Here's how the part is built. I have some questions about the finished solid (model axes, mm). Face numbers are marked on the shaded views. A direction names the side the tool comes from. Give positions to 0.01 mm unless a question says otherwise; leave off trailing zeros. Write each loop counter-clockwise with the first axis right and the second up, starting at its lowest first coordinate (ties: lowest second). Pieces come first, ordered by that corner, then holes. Notation, with made-up numbers: (46, -11) - (69, -11) arc R22 cw to (69, 24) - close; hole circle Ø1 at (57.25, -18.5). An arc over 180 degrees is marked (long way). Write each question's results on one line, items separated by ' | '. Start each with the question number.
Item 1: Suppose I cut it at A-A on z = 0. List the corners of the cut face in (x, y) for me.
Item 2: Will these pins go through, and if not, where does the flat tip stop? P1, Ø2.5, axis at x = -38.89, z = -38.89, coming from the +Y side; P2, Ø4, axis at x = 38.89, z = 38.89, coming from the +Y side; P3, Ø10, axis at y = 26.5, z = 17, coming from the -X side; P4, Ø1, axis at y = 8.5, z = 26, coming from the -X side.
Item 3: Suppose I cut it at B-B on y = 12.5. List the corners of the cut face in (x, z) for me, then the cut area to 3 significant figures.
Item 4: Please list where these lines run through material, in increasing order: line 1 along Z through (x, y) = (0, 25.5); line 2 along Z through (x, y) = (11.5, 15.5); line 3 along Y through (x, z) = (44, 23.5).
Item 5: Which directions (+Z, -Z, +X, -X, +Y, -Y) give clear straight access to the entire face, cutting with the end or side of a thin tool? Please do the marked faces 1 and 2.
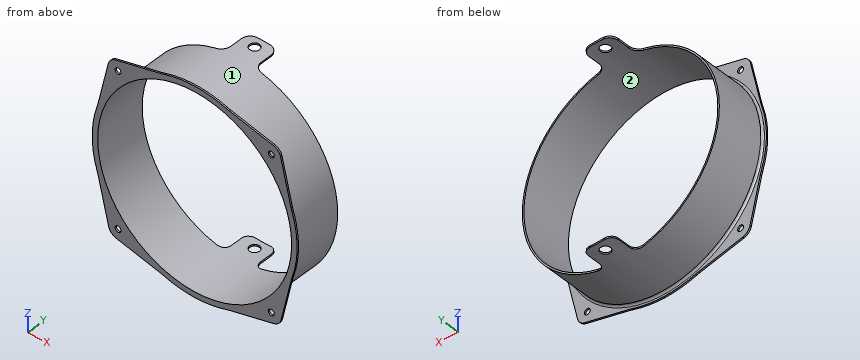
```python
from build123d import *

# Parameters (mm, degrees)
SKETCH1_R               = 50
SKETCH1_R_2             = 1.5
BOSS_EXTRUDE1_DEPTH     = 0.8
SKETCH1_4_R             = 50
SKETCH1_4_R_2           = 49.2
BOSS_EXTRUDE3_DEPTH     = 40
FILLET1_R               = 1
CUT_EXTRUDE1_START      = -14
CUT_EXTRUDE1_DEPTH      = 14
CUT_EXTRUDE2_START      = -14
CUT_EXTRUDE2_DEPTH      = 14
FILLET2_R               = 4
FILLET4_R               = 4
CUT_EXTRUDE3_DEPTH      = 84.713798194
CUT_EXTRUDE3_DEPTH_BACK = 84.713798194
SKETCH16_R              = 2.5


with BuildPart() as part:
    # Sketch1 → Boss-Extrude1 (new body)
    with BuildSketch(Plane(origin=(0, 0, 0), x_dir=(1, 0, 0), z_dir=(0, 1, 0))):
        with BuildLine():
            Line((17.897079586, 48.929734976), (40.149284407, 43.651218265))
            ThreePointArc((40.149284407, 43.651218265), (42.540265174, 42.312242187), (43.866371506, 39.91409958))
            Line((43.866371506, 39.91409958), (49.02521675, 17.633846579))
            ThreePointArc((49.02521675, 17.633846579), (49.23478351, 16.809026698), (49.479249782, 15.993868858))
            ThreePointArc((49.479249782, 15.993868858), (51.999812242, -0.139738387), (49.392575566, -16.259565766))
            ThreePointArc((49.392575566, -16.259565766), (49.143731732, -17.073397941), (48.929734976, -17.897079586))
            Line((48.929734976, -17.897079586), (43.651218265, -40.149284407))
            ThreePointArc((43.651218265, -40.149284407), (42.312242187, -42.540265174), (39.91409958, -43.866371506))
            Line((39.91409958, -43.866371506), (17.633846579, -49.02521675))
            ThreePointArc((17.633846579, -49.02521675), (16.809026698, -49.23478351), (15.993868858, -49.479249782))
            ThreePointArc((15.993868858, -49.479249782), (-0.139738387, -51.999812242), (-16.259565766, -49.392575566))
            ThreePointArc((-16.259565766, -49.392575566), (-17.073397941, -49.143731732), (-17.897079586, -48.929734976))
            Line((-17.897079586, -48.929734976), (-40.149284407, -43.651218265))
            ThreePointArc((-40.149284407, -43.651218265), (-42.540265174, -42.312242187), (-43.866371506, -39.91409958))
            Line((-43.866371506, -39.91409958), (-49.02521675, -17.633846579))
            ThreePointArc((-49.02521675, -17.633846579), (-49.23478351, -16.809026698), (-49.479249782, -15.993868858))
            ThreePointArc((-49.479249782, -15.993868858), (-51.999812242, 0.139738387), (-49.392575566, 16.259565766))
            ThreePointArc((-49.392575566, 16.259565766), (-49.143731732, 17.073397941), (-48.929734976, 17.897079586))
            Line((-48.929734976, 17.897079586), (-43.651218265, 40.149284407))
            ThreePointArc((-43.651218265, 40.149284407), (-42.312242187, 42.540265174), (-39.91409958, 43.866371506))
            Line((-39.91409958, 43.866371506), (-17.633846579, 49.02521675))
            ThreePointArc((-17.633846579, 49.02521675), (-16.809026698, 49.23478351), (-15.993868858, 49.479249782))
            ThreePointArc((-15.993868858, 49.479249782), (-8.026622704, 51.3767781), (0.139738387, 51.999812242))
            ThreePointArc((0.139738387, 51.999812242), (8.302633013, 51.332896714), (16.259565766, 49.392575566))
            ThreePointArc((16.259565766, 49.392575566), (17.073397941, 49.143731732), (17.897079586, 48.929734976))
        make_face()
        with Locations(Location((0, 0, 0), (0, 0, 270))):
            Circle(SKETCH1_R, mode=Mode.SUBTRACT)
        with Locations(Location((-38.8907, 38.8907, 0), (0, 0, 270))):
            Circle(SKETCH1_R_2, mode=Mode.SUBTRACT)
        with Locations(Location((38.8907, 38.8907, 0), (0, 0, 90))):
            Circle(SKETCH1_R_2, mode=Mode.SUBTRACT)
        with Locations(Location((38.8907, -38.8907, 0), (0, 0, 270))):
            Circle(SKETCH1_R_2, mode=Mode.SUBTRACT)
        with Locations(Location((-38.8907, -38.8907, 0), (0, 0, 90))):
            Circle(SKETCH1_R_2, mode=Mode.SUBTRACT)
    extrude(amount=BOSS_EXTRUDE1_DEPTH)

    # Sketch1_4 → Boss-Extrude3 (add)
    with BuildSketch(Plane(origin=(0, 0, 0), x_dir=(1, 0, 0), z_dir=(0, 1, 0))):
        with Locations(Location((0, 0, 0), (0, 0, 270))):
            Circle(SKETCH1_4_R)
        with Locations(Location((0, 0, 0), (0, 0, 270))):
            Circle(SKETCH1_4_R_2, mode=Mode.SUBTRACT)
    extrude(amount=BOSS_EXTRUDE3_DEPTH)

    # Fillet1
    fillet1_edges = [part.edges().sort_by_distance(p)[0] for p in [
        (0, 0.8, -50),
    ]]
    fillet(fillet1_edges, radius=FILLET1_R)

    # Sketch10 → Cut-Extrude1 (cut)
    with BuildSketch(Plane(origin=(0, 40, 0), x_dir=(1, 0, 0), z_dir=(0, 1, 0)).offset(CUT_EXTRUDE1_START)):
        with BuildLine():
            Line((0, 0), (-7.621909697, 49.41565028))
            ThreePointArc((-7.621909697, 49.41565028), (-50, 0), (-7.621909697, -49.41565028))
            Line((-7.621909697, -49.41565028), (0, 0))
        make_face()
    extrude(amount=CUT_EXTRUDE1_DEPTH, mode=Mode.SUBTRACT)

    # Sketch11 → Cut-Extrude2 (cut)
    with BuildSketch(Plane(origin=(0, 40, 0), x_dir=(1, 0, 0), z_dir=(0, 1, 0)).offset(CUT_EXTRUDE2_START)):
        with BuildLine():
            Line((0, 0), (7.621909697, 49.41565028))
            ThreePointArc((7.621909697, 49.41565028), (50, 0), (7.621909697, -49.41565028))
            Line((7.621909697, -49.41565028), (0, 0))
        make_face()
    extrude(amount=CUT_EXTRUDE2_DEPTH, mode=Mode.SUBTRACT)

    # Fillet2
    fillet2_edges = [part.edges().sort_by_distance(p)[0] for p in [
        (-7.560934419, 26, 49.020325078),
        (-7.560934419, 26, -49.020325078),
        (7.560934419, 26, 49.020325078),
        (7.560934419, 26, -49.020325078),
    ]]
    fillet(fillet2_edges, radius=FILLET2_R)

    # Fillet4
    fillet4_edges = [part.edges().sort_by_distance(p)[0] for p in [
        (-7.560934419, 40, -49.020325078),
        (-7.560934419, 40, 49.020325078),
        (7.560934419, 40, 49.020325078),
        (7.560934419, 40, -49.020325078),
    ]]
    fillet(fillet4_edges, radius=FILLET4_R)

    # Sketch16 → Cut-Extrude3 (cut, two sides: drawn at the far end of the back side and taken through both)
    with BuildSketch(Plane.XY.offset(-CUT_EXTRUDE3_DEPTH_BACK)):
        with Locations((0, 35)):
            Circle(SKETCH16_R)
    extrude(amount=CUT_EXTRUDE3_DEPTH + CUT_EXTRUDE3_DEPTH_BACK, mode=Mode.SUBTRACT)


solid = part.part
```
Checked values:
1) outline: (-52, 0) - (-49.2, 0) - (-49.2, 26) - (-50, 26) - (-50, 1.8) arc R1 cw to (-51, 0.8) - (-52, 0.8) - close; (49.2, 0) - (52, 0) - (52, 0.8) - (51, 0.8) arc R1 cw to (50, 1.8) - (50, 26) - (49.2, 26) - close
2) P1: passes through | P2: stops at y = 0.8 | P3: stops at x = -48.53 | P4: stops at x = -43.01
3) outline: circle Ø100 at (0, 0); hole circle Ø98.4 at (0, 0) | area: 249 mm^2
4) line 1: z = -50 to -49.2, 49.2 to 50 | line 2: z = -48.66 to -47.84, 47.84 to 48.66 | line 3: y = 0 to 26
5) face 1: +Y | face 2: +Y, -Y
